from build123d import *

# Parameters (mm, degrees)
FLANGE_BASE1_START                    = -6.35
FLANGE_BASE1_OUTLINE_W                = 300
FLANGE_BASE1_OUTLINE_H                = 248
FLANGE_BASE1_DEPTH                    = 12.7
QUEBRA_CANTO1_START                   = -6.35
QUEBRA_CANTO1_DEPTH                   = 12.7
FURO_ROSCADO_DE_M10X1_52_D            = 8.5
FURO_ROSCADO_DE_M10X1_52_DEPTH        = 29.946342369
FURO_ROSCADO_DE_M10X1_52_TIP          = 2.553657631
ESBO_O11_R                            = 16.5
CORTE_EXTRUS_O1_DEPTH                 = 196.031510275
ESBO_O12_R                            = 37
CORTE_EXTRUS_O2_DEPTH                 = 196.031510275
FURO_ROSCADO_DE_M6X1_01_D             = 5
CORTE_EXTRUS_O5_DEPTH                 = 12.7
ESCAREADO_PARA_SFHCS_M101_D           = 10.5
ESCAREADO_PARA_SFHCS_M101_DEPTH       = 32.5
ESCAREADO_PARA_SFHCS_M101_CSINK_D     = 22.4
ESCAREADO_PARA_SFHCS_M101_CSINK_ANGLE = 90
ESCAREADO_PARA_SFHCS_M101_TIP         = 3.15451825


# Read off the part's stored shape, not the designer's step: Flange-base1, Quebra-Canto1
with BuildPart() as part:
    # Flange-base1 outline → Flange-base1 (new body)
    with BuildSketch(Plane.XY.offset(FLANGE_BASE1_START)):
        Rectangle(FLANGE_BASE1_OUTLINE_W, FLANGE_BASE1_OUTLINE_H)
    extrude(amount=FLANGE_BASE1_DEPTH)

    # Quebra-Canto1 outline → Quebra-Canto1 (cut)
    with BuildSketch(Plane.XY.offset(QUEBRA_CANTO1_START)):
        Polygon((-150, 124), (-150, 109), (-135, 124), align=None)
        Polygon((150, 124), (135, 124), (150, 109), align=None)
    extrude(amount=QUEBRA_CANTO1_DEPTH, mode=Mode.SUBTRACT)

    # Furo roscado de M10x1.52
    with Locations(Plane.XY.offset(6.35)):
        with Locations((-40, 99), (-120, 99), (40, 99), (120, 99)):
            Hole(FURO_ROSCADO_DE_M10X1_52_D / 2, depth=FURO_ROSCADO_DE_M10X1_52_DEPTH)
            with Locations((0, 0, -(FURO_ROSCADO_DE_M10X1_52_DEPTH + FURO_ROSCADO_DE_M10X1_52_TIP / 2))):  # 118° drill point
                Cone(0, FURO_ROSCADO_DE_M10X1_52_D / 2, FURO_ROSCADO_DE_M10X1_52_TIP, mode=Mode.SUBTRACT)

    # Esboço11 → Corte-extrusão1 (cut, through all)
    with BuildSketch(Plane.XY.offset(6.35)):
        with Locations((87.5, -57.664450339)):
            Circle(ESBO_O11_R)
    extrude(amount=-CORTE_EXTRUS_O1_DEPTH, mode=Mode.SUBTRACT)

    # Esboço12 → Corte-extrusão2 (cut, through all)
    with BuildSketch(Plane(origin=(0, 0, -6.35), x_dir=(-1, 0, 0), z_dir=(0, 0, -1))):
        with Locations((-87.5, -57.664450339)):
            Circle(ESBO_O12_R)
    extrude(amount=-CORTE_EXTRUS_O2_DEPTH, mode=Mode.SUBTRACT)

    # Furo roscado de M6x1.01 (through all)
    with Locations(Plane(origin=(0, 0, -6.35), x_dir=(-1, 0, 0), z_dir=(0, 0, -1))):
        with Locations((-122.25, -22.914450339), (-87.5, -57.664450339), (-52.75, -92.414450339), (-52.75, -22.914450339), (-122.25, -92.414450339)):
            Hole(FURO_ROSCADO_DE_M6X1_01_D / 2)

    # Esboço20 → Corte-extrusão5 (cut)
    with BuildSketch(Plane.XY.offset(6.35)):
        with BuildLine():
            Line((-2.5, -14.164450339), (-77.5, -14.164450339))
            ThreePointArc((-77.5, -14.164450339), (-84, -7.664450339), (-77.5, -1.164450339))
            Line((-77.5, -1.164450339), (-2.5, -1.164450339))
            ThreePointArc((-2.5, -1.164450339), (4, -7.664450339), (-2.5, -14.164450339))
        make_face()
    extrude(amount=-CORTE_EXTRUS_O5_DEPTH, mode=Mode.SUBTRACT)

    # Escareado para SFHCS M101
    with Locations(Plane.XY.offset(6.35)):
        with Locations((-130, 70), (-43.333333333, 70), (43.333333333, 70), (130, 70)):
            CounterSinkHole(ESCAREADO_PARA_SFHCS_M101_D / 2, ESCAREADO_PARA_SFHCS_M101_CSINK_D / 2, depth=ESCAREADO_PARA_SFHCS_M101_DEPTH, counter_sink_angle=ESCAREADO_PARA_SFHCS_M101_CSINK_ANGLE)
            with Locations((0, 0, -(ESCAREADO_PARA_SFHCS_M101_DEPTH + ESCAREADO_PARA_SFHCS_M101_TIP / 2))):  # 118° drill point
                Cone(0, ESCAREADO_PARA_SFHCS_M101_D / 2, ESCAREADO_PARA_SFHCS_M101_TIP, mode=Mode.SUBTRACT)


solid = part.part
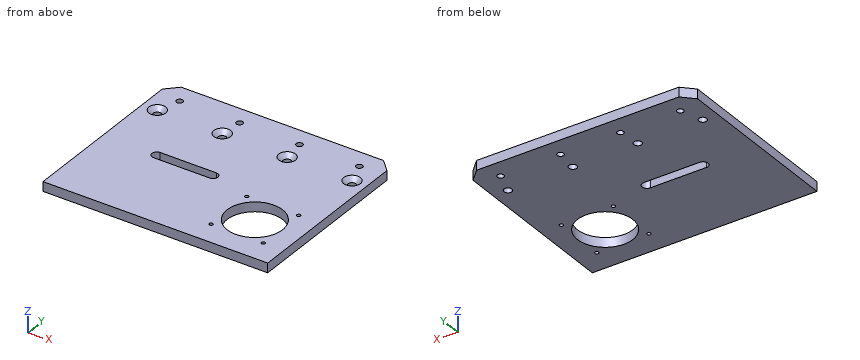
Source: CAD feature listing. Evaluate the final solid. Frame: model axes, mm. Coordinates: 2 decimals unless noted, no trailing zeros. Order: outer loops, then holes, each group sorted by start corner. A loop starts at its lowest first (then second) coordinate and runs counter-clockwise, first axis right, second up. Notation, with made-up numbers: M 26,-24 L 65,-24 A19 ccw 65,3 Z; hole C 50.5,-13 d6. An arc over 180 degrees is marked long. Write each question's results on one line, items separated by ' | '. Start each with the question number.
1. Section C-C, the plane z = -2. State how many separate pieces and enclosed holes the cut face has, then the cut area to 3 significant figures.
2. Section D-D, the plane y = -81. Return the cut outline in (x, z).
3. Material intervals for L1, parallel to Y at x = -42.5, z = -0.75; L2, parallel to Y at x = -23.5, z = -2.25; L3, parallel to X at y = 73.5, z = 0.5, sorted ascending.
4. Pin query (flat end, axial travel): pin 1 (5 mm diameter, centred on x = -40, y = 99, fed in from +Z); pin 2 (13.5 mm diameter, centred on x = -130, y = 70, fed in from +Z); pin 3 (12 mm diameter, centred on x = -43.33, y = 70, fed in from +Z). Return the tip coordinate at first contact, or that it passes through.
5. Section A-A, the plane x = -70.5. Return the cut outline in (y, z).
6. Section B-B, the plane y = 70. Return the cut outline in (x, z).
Solution:
1) separate pieces: 1 | enclosed holes: 14 | area: 68,100 mm²
2) outline: M -150,-6.35 L 58.79,-6.35 L 58.79,6.35 L -150,6.35 Z; M 116.21,-6.35 L 150,-6.35 L 150,6.35 L 116.21,6.35 Z
3) L1: -124 to -14.16, -1.16 to 64.82, 75.18 to 95.56, 102.44 to 124 | L2: -124 to -14.16, -1.16 to 124 | L3: -150 to -134.05, -125.95 to -47.38, -39.29 to 39.29, 47.38 to 125.95, 134.05 to 150
4) pin 1: through | pin 2: z = 1.9 | pin 3: z = 1.15
5) outline: M -124,-6.35 L -14.16,-6.35 L -14.16,6.35 L -124,6.35 Z; M -1.16,-6.35 L 124,-6.35 L 124,6.35 L -1.16,6.35 Z
6) outline: M -150,-6.35 L -135.25,-6.35 L -135.25,0.4 L -141.2,6.35 L -150,6.35 Z; M -124.75,-6.35 L -48.58,-6.35 L -48.58,0.4 L -54.53,6.35 L -118.8,6.35 L -124.75,0.4 Z; M -38.08,-6.35 L 38.08,-6.35 L 38.08,0.4 L 32.13,6.35 L -32.13,6.35 L -38.08,0.4 Z; M 48.58,-6.35 L 124.75,-6.35 L 124.75,0.4 L 118.8,6.35 L 54.53,6.35 L 48.58,0.4 Z; M 135.25,-6.35 L 150,-6.35 L 150,6.35 L 141.2,6.35 L 135.25,0.4 Z
